Verification items for the finished model (mm, model axes). A direction names the side the tool comes from. Give positions to 0.01 mm unless a question says otherwise; leave off trailing zeros. Write each loop counter-clockwise with the first axis right and the second up, starting at its lowest first coordinate (ties: lowest second). Pieces come first, ordered by that corner, then holes. Notation, with made-up numbers: (-29, -10.75) -> (-24, -10.75) arc R18 ccw to (-24, 2.25) -> close; hole circle Ø2 at (73, 69.25). An arc over 180 degrees is marked (long way). Use one line per item in the form item = value. Start each with the question number.
(1) Section check A-A, the plane x = 0. Record the cut outline in (y, z) (3 decimals), plus the area to 3 significant figures.
(2) Set-up check for faces 4 (the face through (0.165, 3.479, -3.746)), 5 (the face through (3.8, 1, 0)): record each of +Z, -Z, +X, -X, +Y, -Y from which the full face is reachable in a straight line by a thin tool's end or side.
(3) Scan lines: L1, parallel to X at y = 0.45, z = 0 (3 decimals); L2, parallel to Y at x = 3.25, z = 2.75; L3, parallel to X at y = 2.75, z = 0.5. Record each from-to range of solid material in increasing order.
(4) Section check B-B, the plane z = 0. Record the cut outline in (x, y) (3 decimals).
(5) Release check for a two-part mould opening along Y. For faces 1 (the face through (-0.81, 1.01, -1.05)), 2 (the face through (-0.9, 0, -1.2)), 3 (the face through (0, 8, 2.675)) record: pulls with the +Y half, pulls with the -Y half, needs draft (parallel to the pull), parting line crosses it, or undercut.
(6) Depth check by flat-ended pin: pin 1 Ø1.5 at (x, z) = (-1, -0.5) entering from +Y; pin 2 Ø1.5 at (x, y) = (-2.5, 10.5) entering from +Z; pin 3 Ø2.5 at (x, y) = (0, 8) entering from +Z (3 decimals); pin 4 Ø2 at (x, z) = (0, 0) entering from +Y. Enter the tip coordinate at first touch or a pass-through.
(7) Section check D-D, the plane z = 2.25. Record the cut outline in (x, y).
(8) Section check C-C, the plane y = 12.5. Record the cut outline in (x, z) (3 decimals), plus the area to 3 significant figures.
from build123d import *

# Parameters (mm, degrees)
ESQUISSE1_W             = 7.6
ESQUISSE1_H             = 10
BOSS_EXTRU_1_DEPTH      = 2
ESQUISSE2_R             = 3.75
ESQUISSE2_R_2           = 2.5
BOSS_EXTRU_2_DEPTH      = 3
ESQUISSE3_R             = 3.175
ESQUISSE3_R_2           = 2.5
BOSS_EXTRU_3_DEPTH      = 10
ESQUISSE4_R             = 1.325
ENL_V_MAT_EXTRU_1_DEPTH = 15.437451299
ESQUISSE6_R             = 2.54
ENL_V_MAT_EXTRU_3_DEPTH = 0.5


with BuildPart() as part:
    # Esquisse1 → Boss.-Extru.1 (new body)
    with BuildSketch(Plane(origin=(0, 0, 0), x_dir=(1, 0, 0), z_dir=(0, 1, 0))):
        Rectangle(ESQUISSE1_W, ESQUISSE1_H)
    extrude(amount=BOSS_EXTRU_1_DEPTH)

    # Esquisse2 → Boss.-Extru.2 (add)
    with BuildSketch(Plane(origin=(0, 2, 0), x_dir=(1, 0, 0), z_dir=(0, 1, 0))):
        with Locations(Location((0, 0, 0), (0, 0, 270))):
            Circle(ESQUISSE2_R)
        with Locations(Location((0, 0, 0), (0, 0, 270))):
            Circle(ESQUISSE2_R_2, mode=Mode.SUBTRACT)
    extrude(amount=BOSS_EXTRU_2_DEPTH)

    # Esquisse3 → Boss.-Extru.3 (add)
    with BuildSketch(Plane(origin=(0, 5, 0), x_dir=(1, 0, 0), z_dir=(0, 1, 0))):
        with Locations(Location((0, 0, 0), (0, 0, 270))):
            Circle(ESQUISSE3_R)
        with Locations(Location((0, 0, 0), (0, 0, 270))):
            Circle(ESQUISSE3_R_2, mode=Mode.SUBTRACT)
    extrude(amount=BOSS_EXTRU_3_DEPTH)

    # Esquisse4 → Enlèv. mat.-Extru.1 (cut, through all)
    with BuildSketch(Plane(origin=(0, 2, 0), x_dir=(1, 0, 0), z_dir=(0, 1, 0))):
        with Locations(Location((0, 0, 0), (0, 0, 270))):
            Circle(ESQUISSE4_R)
    extrude(amount=-ENL_V_MAT_EXTRU_1_DEPTH, mode=Mode.SUBTRACT)

    # Esquisse6 → Enlèv. mat.-Extru.3 (cut)
    with BuildSketch(Plane.XY.offset(3.175)):
        with Locations((0, 8.2)):
            Circle(ESQUISSE6_R)
    extrude(amount=-ENL_V_MAT_EXTRU_3_DEPTH, mode=Mode.SUBTRACT)


solid = part.part
Completed:
q1.outline = (0, -5) -> (2, -5) -> (2, -3.75) -> (5, -3.75) -> (5, -3.175) -> (15, -3.175) -> (15, -2.5) -> (2, -2.5) -> (2, -1.325) -> (0, -1.325) -> close; (0, 1.325) -> (2, 1.325) -> (2, 2.5) -> (15, 2.5) -> (15, 3.175) -> (10.74, 3.175) -> (10.74, 2.675) -> (5.66, 2.675) -> (5.66, 3.175) -> (5, 3.175) -> (5, 3.75) -> (2, 3.75) -> (2, 5) -> (0, 5) -> close
q1.area = 33.2 mm²
q2.face_4 = +Y
q2.face_5 = +Z, -Z, +X, +Y, -Y
q3.L1 = -3.8 to -1.325, 1.325 to 3.8
q3.L2 = 0 to 2
q3.L3 = -3.72 to -2.45, 2.45 to 3.72
q4.outline = (-3.8, 0) -> (-1.325, 0) -> (-1.325, 2) -> (-2.5, 2) -> (-2.5, 15) -> (-3.175, 15) -> (-3.175, 5) -> (-3.75, 5) -> (-3.75, 2) -> (-3.8, 2) -> close; (1.325, 0) -> (3.8, 0) -> (3.8, 2) -> (3.75, 2) -> (3.75, 5) -> (3.175, 5) -> (3.175, 15) -> (2.5, 15) -> (2.5, 2) -> (1.325, 2) -> close
q5.face_1 = needs draft
q5.face_2 = pulls with the -Y half
q5.face_3 = undercut
q6.pin_1 = 2
q6.pin_2 = 2.65
q6.pin_3 = 2.675
q6.pin_4 = through
q7.outline = (-3.8, 0) -> (3.8, 0) -> (3.8, 2) -> (3, 2) -> (3, 5) -> (2.24, 5) -> (2.24, 15) -> (1.09, 15) -> (1.09, 2) -> (-1.09, 2) -> (-1.09, 15) -> (-2.24, 15) -> (-2.24, 5) -> (-3, 5) -> (-3, 2) -> (-3.8, 2) -> close
q8.outline = circle Ø6.35 at (0, 0); hole circle Ø5 at (0, 0)
q8.area = 12.0 mm²
